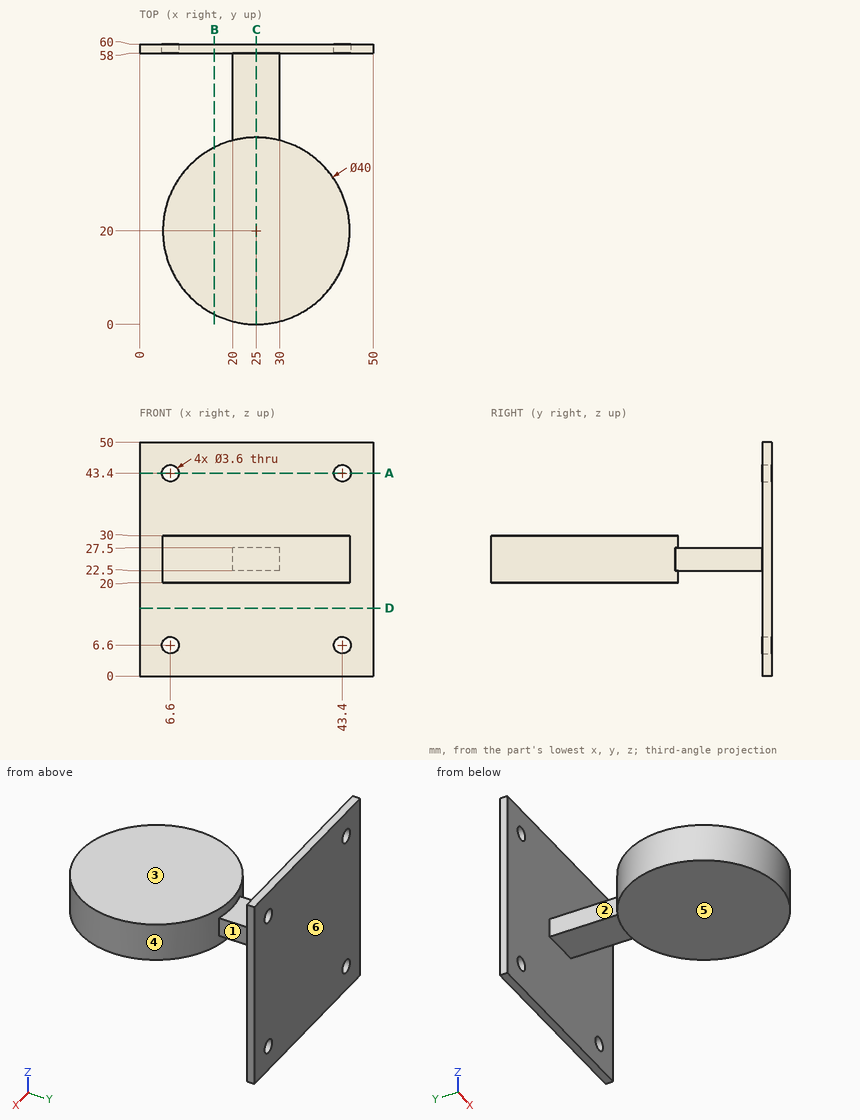
For this review, use the dimensioned drawing (mm, ordinates from the lowest corner) and the shaded views. A direction names the side the tool comes from. Coordinates: 2 decimals unless noted, no trailing zeros. Write each loop counter-clockwise with the first axis right and the second up, starting at its lowest first coordinate (ties: lowest second). Pieces come first, ordered by that corner, then holes. Notation, with made-up numbers: (70.5, 40.25) - (125.5, 40.25) arc R31 ccw to (125.5, 65.25) - close; hole circle Ø2 at (88.25, -18). An arc over 180 degrees is marked (long way). One line per item, written item: value.
1) Add section D-D (z = 14.5). State the section outline as (x, y) points, plus the area to 3 significant figures.
Answer sheet:
outline: (0, 58) - (50, 58) - (50, 60) - (0, 60) - close
area: 100 mm2
2) To check wall thickness, follow probe 1 along Z at (x, y) = (43.4, 58.85); probe 2 along Z at (x, y) = (6, 59). State the ranges of each line that lie inside material, in increasing order.
Answer sheet:
probe 1: z = 0 to 4.8, 8.4 to 41.6, 45.2 to 50
probe 2: z = 0 to 4.9, 8.3 to 41.7, 45.1 to 50
3) For the marked faces 1, 2 and 3, list the 3-axis set-ups (+Z, -Z, +X, -X, +Y, -Y) from which the entire face can be reached by the end or side of a thin tool; tool diameter is ignored.
Answer sheet:
face 1: +Z, -Z, +X
face 2: +Z, -Z, -X
face 3: +Z, +X, -X, -Y
4) Add section A-A (z = 43.4). State the section outline as (x, y) points, plus the area to 3 significant figures.
Answer sheet:
outline: (0, 58) - (4.8, 58) - (4.8, 60) - (0, 60) - close; (8.4, 58) - (41.6, 58) - (41.6, 60) - (8.4, 60) - close; (45.2, 58) - (50, 58) - (50, 60) - (45.2, 60) - close
area: 85.6 mm2
5) Add section B-B (x = 16). State the section outline as (y, z) points, plus the area to 3 significant figures.
Answer sheet:
outline: (2.14, 20) - (37.86, 20) - (37.86, 30) - (2.14, 30) - close; (58, 0) - (60, 0) - (60, 50) - (58, 50) - close
area: 457 mm2
6) Add section C-C (x = 25). State the section outline as (y, z) points.
Answer sheet:
outline: (0, 20) - (40, 20) - (40, 22.5) - (58, 22.5) - (58, 0) - (60, 0) - (60, 50) - (58, 50) - (58, 27.5) - (40, 27.5) - (40, 30) - (0, 30) - close
7) Mouldability with a two-part tool opening along Y and no side actions: class the marked faces 4, 5 and 6 as +Y half, -Y half, draft (parallel to the pull), parting line (faces both ways), or undercut.
Answer sheet:
face 4: undercut
face 5: draft
face 6: +Y half
8) Insertion check: pin 1 (5 mm diameter, centred on x = 25, y = 44, fed in from +Z); pin 2 (2 mm diameter, centred on x = 25.5, y = 39, fed in from -Z); pin 3 (10 mm diameter, centred on y = 48, z = 16.5, fed in from -X); pin 4 (25 mm diameter, centred on x = 34, z = 29, fed in from -Y). Each pin has a flat end and moves straight along its axis. Give the tip position at first contact, or say it passes through.
Answer sheet:
pin 1: stops at z = 27.5
pin 2: stops at z = 20
pin 3: passes through
pin 4: stops at y = 0
